The listing builds one solid part. Answer for the finished solid, in the listing's coordinates (mm). Face numbers are marked on the shaded views. A direction names the side the tool comes from. Round coordinates to 2 decimals unless told otherwise and drop trailing zeros. Order: outer loops, then holes, each group sorted by start corner. A loop starts at its lowest first (then second) coordinate and runs counter-clockwise, first axis right, second up. Notation, with made-up numbers: (-17, -37) - (38, -37) arc R15 ccw to (38, -16) - close; hole circle Ø8 at (65, 2). An arc over 180 degrees is marked (long way). One line per item, written item: value. Start each with the question number.
1. Section B-B, the plane y = 101.5 is taken. Give the vertices of the cut face in (x, z).
2. A tool of negligible diameter and unlimited length cuts with its end or side. For the marked faces 4 and 5, from which of +Z, -Z, +X, -X, +Y, -Y can it reach the whole face along a straight path? Write none if from no direction.
3. Section C-C, the plane x = 1 is taken. Give the vertices of the cut face in (y, z).
4. Section A-A, the plane z = -2.25 is taken. Give the vertices of the cut face in (x, y), then the cut area to 3 significant figures.
5. Straight lines are drawn through the part: line 1 (Z direction, x = 7, y = 162.5); line 2 (X direction, y = 287, z = -11). For each, find the intervals that lie inside material, in ascending order.
6. For a pull along X with two mould halves and no side action, classify the marked faces 1, 2 and 3 as released by +X, released by -X, zero draft, split by the parting line, or undercut.
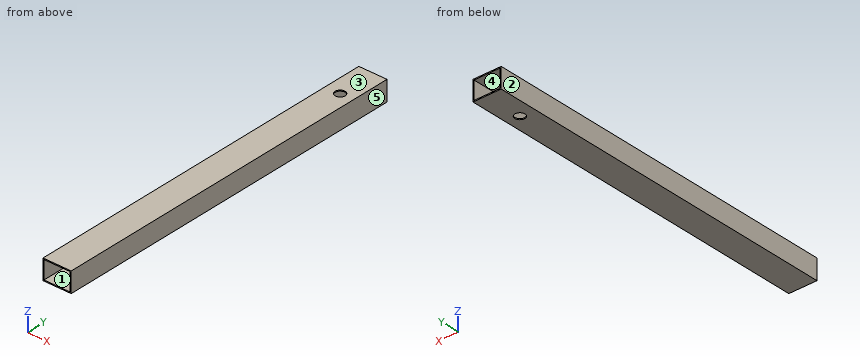
from build123d import *

# Parameters (mm, degrees)
SKETCH1_W           = 35.56
SKETCH1_H           = 25.4
BOSS_EXTRUDE1_DEPTH = 457.2
SKETCH2_W           = 33.02
SKETCH2_H           = 22.86
CUT_EXTRUDE1_DEPTH  = 458.721813332
CUT_EXTRUDE2_REACH  = 460.25
SKETCH3_R           = 6.35
CUT_EXTRUDE3_REACH  = 460.25
SKETCH4_R           = 6.35


with BuildPart() as part:
    # Sketch1 → Boss-Extrude1 (new body)
    with BuildSketch(Plane(origin=(0, 0, 0), x_dir=(1, 0, 0), z_dir=(0, 1, 0))):
        Rectangle(SKETCH1_W, SKETCH1_H)
    extrude(amount=BOSS_EXTRUDE1_DEPTH)

    # Sketch2 → Cut-Extrude1 (cut, through all)
    with BuildSketch(Plane(origin=(0, 457.2, 0), x_dir=(1, 0, 0), z_dir=(0, 1, 0))):
        Rectangle(SKETCH2_W, SKETCH2_H)
    extrude(amount=-CUT_EXTRUDE1_DEPTH, mode=Mode.SUBTRACT)

    # Sketch3 → Cut-Extrude2 (cut, up to next)
    with BuildSketch(Plane.XY.offset(12.7), mode=Mode.PRIVATE) as cut_extrude2_sk1:
        with Locations((0.954776226, 408.643423165)):
            Circle(SKETCH3_R)
    cut_extrude2_tool1 = extrude(cut_extrude2_sk1.sketch, amount=-CUT_EXTRUDE2_REACH, mode=Mode.PRIVATE) & part.part
    add(cut_extrude2_tool1.solids().sort_by_distance((0.954776, 408.643423, 12.7))[0], mode=Mode.SUBTRACT)

    # Sketch4 → Cut-Extrude3 (cut, up to next)
    with BuildSketch(Plane(origin=(0, 0, -12.7), x_dir=(-1, 0, 0), z_dir=(0, 0, -1)), mode=Mode.PRIVATE) as cut_extrude3_sk1:
        with Locations(Location((-0.954776226, 408.643423165, 0), (0, 0, 180))):
            Circle(SKETCH4_R)
    cut_extrude3_tool1 = extrude(cut_extrude3_sk1.sketch, amount=-CUT_EXTRUDE3_REACH, mode=Mode.PRIVATE) & part.part
    add(cut_extrude3_tool1.solids().sort_by_distance((0.954776, 408.643423, -12.7))[0], mode=Mode.SUBTRACT)


solid = part.part
Answer list:
1. outline: (-17.78, -12.7) - (17.78, -12.7) - (17.78, 12.7) - (-17.78, 12.7) - close; hole (-16.51, -11.43) - (16.51, -11.43) - (16.51, 11.43) - (-16.51, 11.43) - close
2. face 4: +Y, -Y
2. face 5: +Z, -Z, +X, +Y, -Y
3. outline: (0, -12.7) - (402.29, -12.7) - (402.29, -11.43) - (0, -11.43) - close; (0, 11.43) - (402.29, 11.43) - (402.29, 12.7) - (0, 12.7) - close; (414.99, -12.7) - (457.2, -12.7) - (457.2, -11.43) - (414.99, -11.43) - close; (414.99, 11.43) - (457.2, 11.43) - (457.2, 12.7) - (414.99, 12.7) - close
4. outline: (-17.78, 0) - (-16.51, 0) - (-16.51, 457.2) - (-17.78, 457.2) - close; (16.51, 0) - (17.78, 0) - (17.78, 457.2) - (16.51, 457.2) - close
4. area: 1,160 mm²
5. line 1: z = -12.7 to -11.43, 11.43 to 12.7
5. line 2: x = -17.78 to -16.51, 16.51 to 17.78
6. face 1: undercut
6. face 2: released by -X
6. face 3: zero draft
